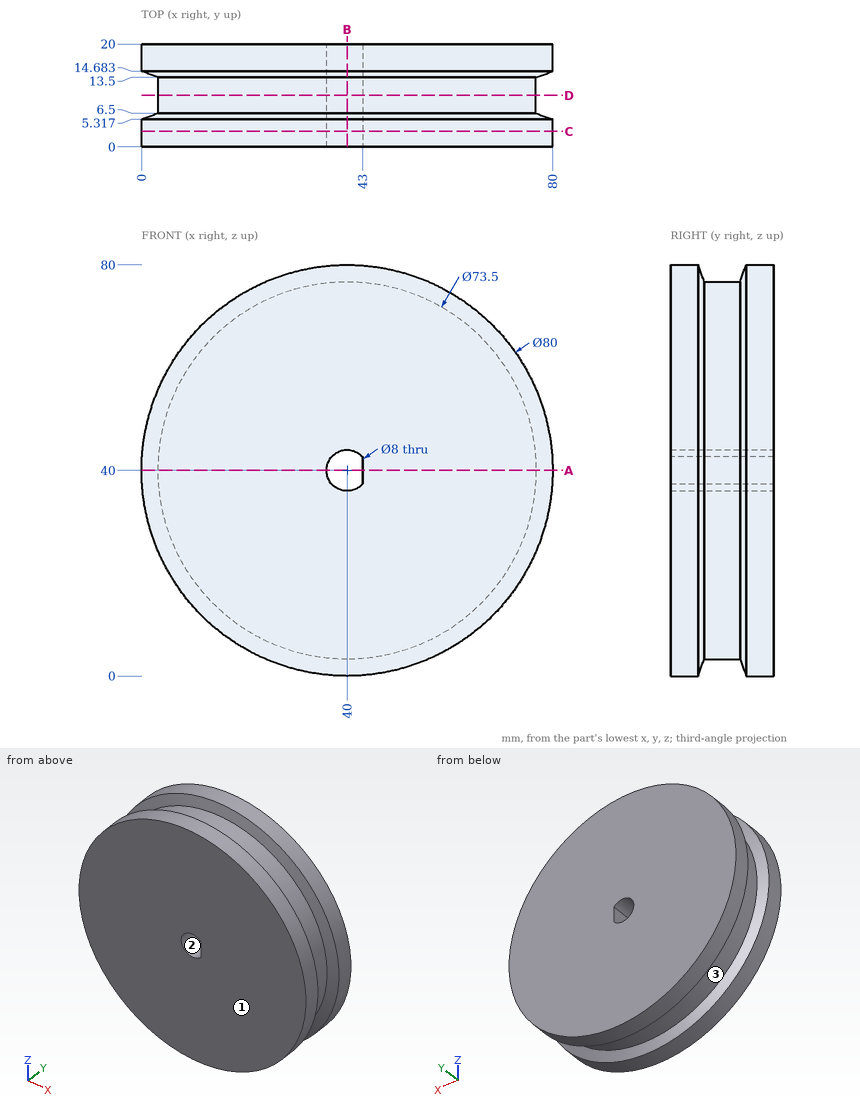
Source: three-view drawing plus pictorial views. Frame: mm from the lowest corner of the part. Give positions to 0.01 mm unless a question says otherwise; leave off trailing zeros. Order: outer loops, then holes, each group sorted by start corner. A loop starts at its lowest first (then second) coordinate and runs counter-clockwise, first axis right, second up. Notation, with made-up numbers: M -20.5,69.25 L 17.5,69.25 A13 cw 17.5,92.25 Z; hole C -7.75,-13 d10. An arc over 180 degrees is marked long. One line per question, with ' | ' between items.
1) Section B-B on x = 40. Output: boundary loops of the cut face in (y, z), and give its area (3 significant figures).
Filled in:
outline: M 0,0 L 5.32,0 L 6.5,3.25 L 13.5,3.25 L 14.68,0 L 20,0 L 20,36 L 0,36 Z; M 0,44 L 20,44 L 20,80 L 14.68,80 L 13.5,76.75 L 6.5,76.75 L 5.32,80 L 0,80 Z | area: 1,390 mm2
2) Section C-C on y = 3. Output: boundary loops of the cut face in (x, z).
Filled in:
outline: C 40,40 d80; hole M 43,37.35 L 43,42.65 A4 ccw long Z
3) Section A-A on z = 40. Output: boundary loops of the cut face in (x, y), and give its area (3 significant figures).
Filled in:
outline: M 0,0 L 36,0 L 36,20 L 0,20 L 0,14.68 L 3.25,13.5 L 3.25,6.5 L 0,5.32 Z; M 43,0 L 80,0 L 80,5.32 L 76.75,6.5 L 76.75,13.5 L 80,14.68 L 80,20 L 43,20 Z | area: 1,410 mm2
4) Contact query for flat-ended pins moving along their axis: P1, Ø2, axis at x = 66.5, y = 3, coming from the +Z side; P2, Ø2, axis at y = 6, z = 50, coming from the +X side; P3, Ø6, axis at y = 6.5, z = 40, coming from the -X side. Output: stop coordinate, or through.
Filled in:
P1: stops at z = 70.82 | P2: stops at x = 78.91 | P3: stops at x = 0
5) Section D-D on y = 10. Output: boundary loops of the cut face in (x, z), and give its area (3 significant figures).
Filled in:
outline: C 40,40 d73.5; hole M 43,37.35 L 43,42.65 A4 ccw long Z | area: 4,200 mm2
6) Draft query along Y for the marked faces 1, 2 and 3. Return one class per face: pulls with the +Y half, pulls with the -Y half, needs draft (parallel to the pull), parting line crosses it, or undercut.
Filled in:
face 1: pulls with the -Y half | face 2: needs draft | face 3: undercut
7) Ray query, L1, parallel to Z at x = 40, y = 13; L2, parallel to Z at x = 40, y = 4.75; L3, parallel to X at y = 10.25, z = 40. Return the intervals inside material, ascending.
Filled in:
L1: z = 3.25 to 36, 44 to 76.75 | L2: z = 0 to 36, 44 to 80 | L3: x = 3.25 to 36, 43 to 76.75
